Check sheet for the modelled part. Datum: model origin and axes. Units: mm. A direction names the side the tool comes from. Give positions to 0.01 mm unless a question says otherwise; leave off trailing zeros. Order: outer loops, then holes, each group sorted by start corner. A loop starts at its lowest first (then second) coordinate and runs counter-clockwise, first axis right, second up. Notation, with made-up numbers: (-2, 77) -> (2, 77) arc R4 cw to (2, 83) -> close; hole circle Ø8 at (53, 12). An arc over 180 degrees is marked (long way). Answer in a Markdown table with one row per item. Add a question column.
(1) Go/stop test with flat-tipped pins: pin 1 (1.5 mm diameter, centred on x = 56, z = 1, fed in from +Y); pin 2 (6 mm diameter, centred on y = 0.5, z = -1, fed in from -X); pin 3 (1.5 mm diameter, centred on x = 14, z = 1, fed in from +Y); pin 4 (1 mm diameter, centred on x = 27, y = 2, fed in from -Z). Record where each tip stops, or that it passes through.
(2) Cross-section at C-C (x = 50.5). Record the cut outline in (y, z).
(3) Cross-section at A-A (z = 0). Record the cut outline in (x, y).
(4) Cross-section at D-D (x = 10). Record the cut outline in (y, z), then the cut area to 3 significant figures.
(5) Thickness scan on L1, parallel to X at y = 4.5, z = -1.75; L2, parallel to X at y = -0.5, z = 5.25; L3, parallel to Y at x = 19, z = -2.5. Record the ranges inside material, lowest first. Write a range as [from, to].
(6) Release check for a two-part mould opening along X. For faces 6 (the face through (13.5, 4.92, -1.36)), 7 (the face through (3.94, 1.49, 4.72)), 8 (the face through (8.49, 4.05, 2.58)) record: released by +X, released by -X, zero draft, split by the parting line, or undercut.
(7) Set-up check for faces 1 (the face through (58.76, 4.05, -2.58)), 2 (the face through (69.77, 1.49, -4.72)), 3 (the face through (11.22, 1.49, 4.72)), 4 (the face through (33, -6, 0)), 5 (the face through (0, 0, 0)): record each of +Z, -Z, +X, -X, +Y, -Y from which the full face is reachable in a straight line by a thin tool's end or side.
Autodesk Inventor part; units mm, degrees
ref_plane "YZ Plane" through (0, 0, 0) normal (1, 0, 0) x (0, 1, 0)
ref_plane "XZ Plane" through (0, 0, 0) normal (0, 1, 0) x (-1, 0, 0)
ref_plane "XY Plane" through (0, 0, 0) normal (0, 0, 1) x (1, 0, 0)
sketch "스케치1" plane through (0, 0, 0) normal (1, 0, 0) x (0, 1, 0)
  circle A0 centre (0, 0) radius 6
  dimension "d0" = 12
extrude "돌출1" add sketch "스케치1" along normal blind 80
sketch "스케치2" plane through (80, 0, 0) normal (1, 0, 0) x (0, 0, -1)
  circle A0 centre (0, 0) radius 6
  circle A1 centre (0, 0) radius 4.95
  dimension "d3" = 9.9
extrude "돌출2" cut sketch "스케치2" against normal blind 26
sketch "스케치3" plane through (80, 0, 0) normal (1, 0, 0) x (0, 0, -1)
  circle A0 centre (0, 0) radius 4.95
  circle A1 centre (0, 0) radius 4.8
  dimension "d6" = 9.9
  dimension "d7" = 9.6
extrude "돌출3" cut sketch "스케치3" against normal blind 21.75
sketch "스케치4" plane through (80, 0, 0) normal (1, 0, 0) x (0, 0, -1)
  circle A0 centre (0, 0) radius 4.95
  circle A1 centre (0, 0) radius 4.8
  dimension "d10" = 9.9
  dimension "d11" = 9.6
extrude "돌출4" add sketch "스케치4" against normal blind 20.75
sketch "스케치5" plane through (0, 0, 0) normal (-1, 0, 0) x (0, 0, 1)
  circle A0 centre (0, 0) radius 6
  circle A1 centre (0, 0) radius 4.95
  dimension "d14" = 12
  dimension "d15" = 9.9
extrude "돌출5" cut sketch "스케치5" against normal blind 13.5
sketch "스케치6" plane through (0, 0, 0) normal (-1, 0, 0) x (0, 0, 1)
  circle A0 centre (0, 0) radius 4.95
  circle A1 centre (0, 0) radius 4.8
  dimension "d18" = 9.9
  dimension "d19" = 9.6
extrude "돌출6" cut sketch "스케치6" against normal blind 9
sketch "스케치7" plane through (0, 0, 0) normal (-1, 0, 0) x (0, 0, 1)
  circle A0 centre (0, 0) radius 4.95
  circle A1 centre (0, 0) radius 4.8
  dimension "d22" = 9.9
  dimension "d23" = 9.6
extrude "돌출7" add sketch "스케치7" against normal blind 8
properties part number "10PI축"
Answer below:
| question | item | result |
|---|---|---|
| 1 | pin 1 | stops at y = 4.94 |
| 1 | pin 2 | stops at x = 0 |
| 1 | pin 3 | stops at y = 5.99 |
| 1 | pin 4 | stops at z = -5.81 |
| 2 | outline | circle Ø12 at (0, 0) |
| 3 | outline | (0, -4.95) -> (8, -4.95) -> (8, -4.8) -> (9, -4.8) -> (9, -4.95) -> (13.5, -4.95) -> (13.5, -6) -> (54, -6) -> (54, -4.95) -> (58.25, -4.95) -> (58.25, -4.8) -> (59.25, -4.8) -> (59.25, -4.95) -> (80, -4.95) -> (80, 4.95) -> (59.25, 4.95) -> (59.25, 4.8) -> (58.25, 4.8) -> (58.25, 4.95) -> (54, 4.95) -> (54, 6) -> (13.5, 6) -> (13.5, 4.95) -> (9, 4.95) -> (9, 4.8) -> (8, 4.8) -> (8, 4.95) -> (0, 4.95) -> close |
| 4 | outline | circle Ø9.9 at (0, 0) |
| 4 | area | 77.0 mm² |
| 5 | L1 | x = [0, 8], [9, 58.25], [59.25, 80] |
| 5 | L2 | x = [13.5, 54] |
| 5 | L3 | y = [-5.45, 5.45] |
| 6 | face 6 | released by -X |
| 6 | face 7 | zero draft |
| 6 | face 8 | undercut |
| 7 | face 1 | none |
| 7 | face 2 | +X |
| 7 | face 3 | -X |
| 7 | face 4 | +X, -X |
| 7 | face 5 | +Z, -Z, -X, +Y, -Y |
